Autodesk Inventor part; units mm, degrees
ref_plane "YZ Plane" through (0, 0, 0) normal (1, 0, 0) x (0, 1, 0)
ref_plane "XZ Plane" through (0, 0, 0) normal (0, 1, 0) x (-1, 0, 0)
ref_plane "XY Plane" through (0, 0, 0) normal (0, 0, 1) x (1, 0, 0)
sketch "Sketch1" plane through (0, 0, 0) normal (0, 1, 0) x (-1, 0, 0)
  circle A0 centre (0, 0) radius 35
extrude "Extrusion1" add sketch "Sketch1" along normal blind 40
sketch "Sketch2" plane through (0, 40, 0) normal (0, 1, 0) x (1, 0, 0)
  circle A0 centre (0, 0) radius 15.5
  dimension "d4" = 31
extrude "Extrusion2" cut sketch "Sketch2" against normal blind 10
sketch "Sketch3" plane through (0, 30, 0) normal (0, 1, 0) x (1, 0, 0)
  circle A0 centre (0, 0) radius 6
  dimension "d7" = 12
extrude "Extrusion3" cut sketch "Sketch3" against normal through all
sketch "Sketch4" plane through (0, 0, 0) normal (0, -1, 0) x (1, 0, 0)
  circle A0 centre (25, 0) radius 3
  point P0 (0, 0)
  dimension "d14" = 6
extrude "Extrusion4" cut sketch "Sketch4" against normal through all
properties part number "Engine"
Could you check a few things on this model? Use its own coordinates, in mm. A direction names the side the tool comes from. Give positions to 0.01 mm unless a question says otherwise; leave off trailing zeros. Write each loop counter-clockwise with the first axis right and the second up, starting at its lowest first coordinate (ties: lowest second). Pieces come first, ordered by that corner, then holes. Notation, with made-up numbers: (48.5, 80.5) -> (87.5, 80.5) arc R17 ccw to (87.5, 97.5) -> close; hole circle Ø4 at (-13, 88.25). An arc over 180 degrees is marked (long way). Answer as a JSON object with one key per item and string values.
Q1. Will these pins go through, and if not, where does the flat tip stop? pin 1 Ø5 at (y, z) = (35.5, 11) entering from -X; pin 2 Ø15.5 at (x, z) = (1, -1) entering from +Y; pin 3 Ø5 at (x, y) = (-4, 9) entering from +Z.
Taken from the geometry:
{"pin 1": "stops at x = -33.95", "pin 2": "stops at y = 30", "pin 3": "stops at z = 34.97"}
Q2. We'd pull the mould along X, two halves only. Please class faces 3 (the flat face through (0, 30, 7)), 4 (the flat face through (-15, 40, -7)), 5 (the cylindrical face through (-6, 15, 0)), 6 (the cylindrical face through (28, 20, 21)): released by +X, released by -X, zero draft, split by the parting line, or undercut.
Taken from the geometry:
{"face 3": "undercut", "face 4": "zero draft", "face 5": "undercut", "face 6": "split by the parting line"}
Q3. Suppose I cut it at D-D on x = 25. Write out the boundary of the cut face in (y, z), then the cut area to 3 significant figures.
Taken from the geometry:
{"outline": "(0, -24.49) -> (40, -24.49) -> (40, -3) -> (0, -3) -> close; (0, 3) -> (40, 3) -> (40, 24.49) -> (0, 24.49) -> close", "area": "1,720 mm²"}
Q4. Suppose I cut it at A-A on z = 0. Write out the boundary of the cut face in (x, y), then the cut area to 3 significant figures.
Taken from the geometry:
{"outline": "(-35, 0) -> (-6, 0) -> (-6, 30) -> (-15.5, 30) -> (-15.5, 40) -> (-35, 40) -> close; (6, 0) -> (22, 0) -> (22, 40) -> (15.5, 40) -> (15.5, 30) -> (6, 30) -> close; (28, 0) -> (35, 0) -> (35, 40) -> (28, 40) -> close", "area": "1,890 mm²"}
Q5. Suppose I cut it at C-C on y = 22.5. Write out the boundary of the cut face in (x, z), then the cut area to 3 significant figures.
Taken from the geometry:
{"outline": "circle Ø70 at (0, 0); hole circle Ø12 at (0, 0); hole circle Ø6 at (25, 0)", "area": "3,710 mm²"}
Q6. Suppose I cut it at B-B on x = 0. Write out the boundary of the cut face in (y, z).
Taken from the geometry:
{"outline": "(0, -35) -> (40, -35) -> (40, -15.5) -> (30, -15.5) -> (30, -6) -> (0, -6) -> close; (0, 6) -> (30, 6) -> (30, 15.5) -> (40, 15.5) -> (40, 35) -> (0, 35) -> close"}
Q7. Please list where these lines run through material, in increasing order: L1, parallel to Z at x = 0, y = 7.75; L2, parallel to Y at x = 13, z = 7; L3, parallel to Z at x = 25, y = 13.
Taken from the geometry:
{"L1": "z = -35 to -6, 6 to 35", "L2": "y = 0 to 30", "L3": "z = -24.49 to -3, 3 to 24.49"}
Q8. Which directions (+Z, -Z, +X, -X, +Y, -Y) give clear straight access to the entire face, cutting with the end or side of a thin tool? Please do faces 1 (the cylindrical face through (-2.018, 35.07, -15.368)), 2 (the cylindrical face through (22, 20, 0)).
Taken from the geometry:
{"face 1": "+Y", "face 2": "+Y, -Y"}
